Can you work these out from the model? Positions are in its coordinate system, mm. A direction names the side the tool comes from. Round coordinates to 2 decimals unless told otherwise and drop trailing zeros. Write each loop counter-clockwise with the first axis right and the second up, starting at its lowest first coordinate (ties: lowest second). Pieces come first, ordered by that corner, then holes. Notation, with made-up numbers: M 56.25,66 L 113.25,66 A15 cw 113.25,71 Z; hole C 42.25,-15.75 d8. An arc over 180 degrees is marked long. Answer as a JSON object with one key per item and string values. Group by question number.
1) Suppose I cut it at B-B, the plane x = 2.5. Write out the boundary of the cut face in (y, z).
2) On a 3-axis mill with a long thin cutter (end or side, diameter ignored), from which of +Z, -Z, +X, -X, +Y, -Y can I reach the whole of each face in a straight line? I mean faces 1 (the cylindrical face through (-5.416, 0.986, -0.011)), 2 (the flat face through (-13, 0, 2)), 3 (the flat face through (17, 1, 0)), 4 (the flat face through (7.5, -1, 0)). Say none if no direction works.
3) Please list where these lines run through material, in increasing order: L1, parallel to X at y = 1.4, z = 0; L2, parallel to X at y = -1.7, z = 2.5; L3, parallel to Y at x = -7, z = 3.75. Write a range as [from, to].
4) I'm going to push flat-ended pins straight in: pin 1 Ø4.5 at (x, z) = (-13.5, 0) entering from -Y; pin 2 Ø1 at (y, z) = (-1.5, -2) entering from +X; pin 3 Ø0.6 at (y, z) = (-1, -3) entering from -X. Where does each tip first touch, or does it pass through?
5) Suppose I cut it at D-D, the plane y = 0.7. State how many separate pieces and enclosed holes the cut face has, and give its area (3 significant figures).
6) Suppose I cut it at C-C, the plane z = -2.25. Write out the boundary of the cut face in (x, y), and give its area (3 significant figures).
7) Suppose I cut it at A-A, the plane z = 0. Write out the boundary of the cut face in (x, y).
from build123d import *

# Parameters (mm, degrees)
SKETCH1_W           = 34
SKETCH1_H           = 16
SKETCH1_R           = 1.75
BOSS_EXTRUDE1_DEPTH = 2
SKETCH1_3_W         = 2.5
SKETCH1_3_H         = 16
BOSS_EXTRUDE2_DEPTH = 2
CUT_EXTRUDE2_DEPTH  = 19.894443628
FILLET1_SIZE        = 6
FILLET1_SIZE_2      = 3
FILLET2_SIZE        = 6
FILLET2_SIZE_2      = 3


with BuildPart() as part:
    # Sketch1 → Boss-Extrude1 (new body)
    with BuildSketch(Plane(origin=(0, 0, 0), x_dir=(1, 0, 0), z_dir=(0, 1, 0))):
        Rectangle(SKETCH1_W, SKETCH1_H)
        with Locations(Location((-13.5, 0, 0), (0, 0, 270))):
            Circle(SKETCH1_R, mode=Mode.SUBTRACT)
        with Locations(Location((13.5, 0, 0), (0, 0, 270))):
            Circle(SKETCH1_R, mode=Mode.SUBTRACT)
    extrude(amount=BOSS_EXTRUDE1_DEPTH)

    # Sketch1<3> → Boss-Extrude2 (add)
    with BuildSketch(Plane(origin=(0, 0, 0), x_dir=(1, 0, 0), z_dir=(0, 1, 0))):
        with Locations((-8.75, 0)):
            Rectangle(SKETCH1_3_W, SKETCH1_3_H)
        with Locations((8.75, 0)):
            Rectangle(SKETCH1_3_W, SKETCH1_3_H)
    extrude(amount=-BOSS_EXTRUDE2_DEPTH)

    # Sketch2 → Cut-Extrude2 (cut, through all)
    with BuildSketch(Plane.XZ):
        with BuildLine():
            ThreePointArc((-5.145390176, -0.683941129), (-5.415852972, 0), (-5.145390176, 0.683941129))
            Line((-5.145390176, 0.683941129), (-0.729537204, 5.394184299))
            ThreePointArc((-0.729537204, 5.394184299), (0, 5.71024317), (0.729537204, 5.394184299))
            Line((0.729537204, 5.394184299), (5.145390176, 0.683941129))
            ThreePointArc((5.145390176, 0.683941129), (5.415852972, 0), (5.145390176, -0.683941129))
            Line((5.145390176, -0.683941129), (0.729537204, -5.394184299))
            ThreePointArc((0.729537204, -5.394184299), (0, -5.71024317), (-0.729537204, -5.394184299))
            Line((-0.729537204, -5.394184299), (-5.145390176, -0.683941129))
        make_face()
    extrude(amount=-CUT_EXTRUDE2_DEPTH, mode=Mode.SUBTRACT)

    # Fillet1
    # an asymmetric fillet: 6, 3 mm, written as the material it takes off along each edge
    with BuildSketch(Plane(origin=(17, -15, 8), x_dir=(-1, 0, 0), z_dir=(0, 1, 0))) as fillet1_piece_1:
        with BuildLine():
            Bezier((FILLET1_SIZE, 0), (0, 0), (0, -FILLET1_SIZE_2), weights=[1, 0.707106781, 1])
            Line((0, -FILLET1_SIZE_2), (0, 0))
            Line((0, 0), (FILLET1_SIZE, 0))
        make_face()
    extrude(amount=32, mode=Mode.SUBTRACT)
    with BuildSketch(Plane(origin=(-17, -15, -8), x_dir=(0, 0, 1), z_dir=(0, 1, 0))) as fillet1_piece_2:
        with BuildLine():
            Bezier((FILLET1_SIZE_2, 0), (0, 0), (0, FILLET1_SIZE), weights=[1, 0.707106781, 1])
            Line((0, FILLET1_SIZE), (0, 0))
            Line((0, 0), (FILLET1_SIZE_2, 0))
        make_face()
    extrude(amount=32, mode=Mode.SUBTRACT)

    # Fillet2
    # an asymmetric fillet: 6, 3 mm, written as the material it takes off along each edge
    with BuildSketch(Plane(origin=(17, -15, -8), x_dir=(-1, 0, 0), z_dir=(0, 1, 0)), Plane(origin=(-17, -15, 8), x_dir=(1, 0, 0), z_dir=(0, 1, 0))) as fillet2_piece_1:
        with BuildLine():
            Bezier((FILLET2_SIZE, 0), (0, 0), (0, FILLET2_SIZE_2), weights=[1, 0.707106781, 1])
            Line((0, FILLET2_SIZE_2), (0, 0))
            Line((0, 0), (FILLET2_SIZE, 0))
        make_face()
    extrude(amount=32, mode=Mode.SUBTRACT)


solid = part.part
Results:
{
 "1": {"outline": "M 0,-8 L 2,-8 L 2,-3.51 L 0,-3.51 Z; M 0,3.51 L 2,3.51 L 2,8 L 0,8 Z"},
 "2": {"face 1": "+Y, -Y", "face 2": "+Z, -Z, -X, -Y", "face 3": "+Z, -Z, +X, +Y, -Y", "face 4": "+Z, -Z, -Y"},
 "3": {"L1": "[-17, -15.25], [-11.75, -5.42], [5.42, 11.75], [15.25, 17]", "L2": "[-10, -7.5], [7.5, 10]", "L3": "[0, 2]"},
 "4": {"pin 1": "y = 0", "pin 2": "x = 10", "pin 3": "x = -10"},
 "5": {"separate pieces": "1", "enclosed holes": "3", "area": "439 mm^2"},
 "6": {"outline": "M -17,0 L -10,0 L -10,-2 L -7.5,-2 L -7.5,0 L -3.68,0 L -3.68,2 L -17,2 Z; M 3.68,0 L 7.5,0 L 7.5,-2 L 10,-2 L 10,0 L 17,0 L 17,2 L 3.68,2 Z", "area": "63.3 mm^2"},
 "7": {"outline": "M -17,0 L -15.25,0 L -15.25,2 L -17,2 Z; M -11.75,0 L -10,0 L -10,-2 L -7.5,-2 L -7.5,0 L -5.42,0 L -5.42,2 L -11.75,2 Z; M 5.42,0 L 7.5,0 L 7.5,-2 L 10,-2 L 10,0 L 11.75,0 L 11.75,2 L 5.42,2 Z; M 15.25,0 L 17,0 L 17,2 L 15.25,2 Z"}
}
